from build123d import *

# Parameters (mm, degrees)
SKETCH1_R          = 3.4036
EXTRUDE1_DEPTH     = 1219.2
CUT_EXTRUDE1_DEPTH = 1221.019934263


with BuildPart() as part:
    # Sketch1 → Extrude1 (new, symmetric)
    with BuildSketch(Plane.XY):
        with BuildLine():
            Line((-20, 16.952), (-20, 4.7625))
            ThreePointArc((-20, 4.7625), (-19.776815367, 4.223684633), (-19.238, 4.0005))
            Line((-19.238, 4.0005), (-16.2662, 4.0005))
            ThreePointArc((-16.2662, 4.0005), (-15.727384633, 4.223684633), (-15.5042, 4.7625))
            Line((-15.5042, 4.7625), (-15.5042, 10.485558599))
            ThreePointArc((-15.5042, 10.485558599), (-15.033804775, 11.189554802), (-14.203384633, 11.024373966))
            Line((-14.203384633, 11.024373966), (-8.635059555, 5.456048889))
            ThreePointArc((-8.635059555, 5.456048889), (-7.985348265, 4.483687227), (-7.7572, 3.336708444))
            Line((-7.7572, 3.336708444), (-7.7572, -3.336708444))
            ThreePointArc((-7.7572, -3.336708444), (-7.985348265, -4.483687227), (-8.635059555, -5.456048889))
            Line((-8.635059555, -5.456048889), (-14.203384633, -11.024373966))
            ThreePointArc((-14.203384633, -11.024373966), (-15.033804775, -11.189554802), (-15.5042, -10.485558599))
            Line((-15.5042, -10.485558599), (-15.5042, -4.7625))
            ThreePointArc((-15.5042, -4.7625), (-15.727384633, -4.223684633), (-16.2662, -4.0005))
            Line((-16.2662, -4.0005), (-19.238, -4.0005))
            ThreePointArc((-19.238, -4.0005), (-19.776815367, -4.223684633), (-20, -4.7625))
            Line((-20, -4.7625), (-20, -16.952))
            ThreePointArc((-20, -16.952), (-19.107261469, -19.107261469), (-16.952, -20))
            Line((-16.952, -20), (-4.7625, -20))
            ThreePointArc((-4.7625, -20), (-4.223684633, -19.776815367), (-4.0005, -19.238))
            Line((-4.0005, -19.238), (-4.0005, -16.2662))
            ThreePointArc((-4.0005, -16.2662), (-4.223684633, -15.727384633), (-4.7625, -15.5042))
            Line((-4.7625, -15.5042), (-10.485558599, -15.5042))
            ThreePointArc((-10.485558599, -15.5042), (-11.189554802, -15.033804775), (-11.024373966, -14.203384633))
            Line((-11.024373966, -14.203384633), (-5.456048889, -8.635059555))
            ThreePointArc((-5.456048889, -8.635059555), (-4.483687227, -7.985348265), (-3.336708444, -7.7572))
            Line((-3.336708444, -7.7572), (3.336708444, -7.7572))
            ThreePointArc((3.336708444, -7.7572), (4.483687227, -7.985348265), (5.456048889, -8.635059555))
            Line((5.456048889, -8.635059555), (11.024373966, -14.203384633))
            ThreePointArc((11.024373966, -14.203384633), (11.189554802, -15.033804775), (10.485558599, -15.5042))
            Line((10.485558599, -15.5042), (4.7625, -15.5042))
            ThreePointArc((4.7625, -15.5042), (4.223684633, -15.727384633), (4.0005, -16.2662))
            Line((4.0005, -16.2662), (4.0005, -19.238))
            ThreePointArc((4.0005, -19.238), (4.223684633, -19.776815367), (4.7625, -20))
            Line((4.7625, -20), (16.952, -20))
            ThreePointArc((16.952, -20), (19.107261469, -19.107261469), (20, -16.952))
            Line((20, -16.952), (20, -4.7625))
            ThreePointArc((20, -4.7625), (19.776815367, -4.223684633), (19.238, -4.0005))
            Line((19.238, -4.0005), (16.2662, -4.0005))
            ThreePointArc((16.2662, -4.0005), (15.727384633, -4.223684633), (15.5042, -4.7625))
            Line((15.5042, -4.7625), (15.5042, -10.485558599))
            ThreePointArc((15.5042, -10.485558599), (15.033804775, -11.189554802), (14.203384633, -11.024373966))
            Line((14.203384633, -11.024373966), (8.635059555, -5.456048889))
            ThreePointArc((8.635059555, -5.456048889), (7.985348265, -4.483687227), (7.7572, -3.336708444))
            Line((7.7572, -3.336708444), (7.7572, 3.336708444))
            ThreePointArc((7.7572, 3.336708444), (7.985348265, 4.483687227), (8.635059555, 5.456048889))
            Line((8.635059555, 5.456048889), (14.203384633, 11.024373966))
            ThreePointArc((14.203384633, 11.024373966), (15.033804775, 11.189554802), (15.5042, 10.485558599))
            Line((15.5042, 10.485558599), (15.5042, 4.7625))
            ThreePointArc((15.5042, 4.7625), (15.727384633, 4.223684633), (16.2662, 4.0005))
            Line((16.2662, 4.0005), (19.238, 4.0005))
            ThreePointArc((19.238, 4.0005), (19.776815367, 4.223684633), (20, 4.7625))
            Line((20, 4.7625), (20, 16.952))
            ThreePointArc((20, 16.952), (19.107261469, 19.107261469), (16.952, 20))
            Line((16.952, 20), (4.7625, 20))
            ThreePointArc((4.7625, 20), (4.223684633, 19.776815367), (4.0005, 19.238))
            Line((4.0005, 19.238), (4.0005, 16.2662))
            ThreePointArc((4.0005, 16.2662), (4.223684633, 15.727384633), (4.7625, 15.5042))
            Line((4.7625, 15.5042), (10.485558599, 15.5042))
            ThreePointArc((10.485558599, 15.5042), (11.189554802, 15.033804775), (11.024373966, 14.203384633))
            Line((11.024373966, 14.203384633), (5.456048889, 8.635059555))
            ThreePointArc((5.456048889, 8.635059555), (4.483687227, 7.985348265), (3.336708444, 7.7572))
            Line((3.336708444, 7.7572), (-3.336708444, 7.7572))
            ThreePointArc((-3.336708444, 7.7572), (-4.483687227, 7.985348265), (-5.456048889, 8.635059555))
            Line((-5.456048889, 8.635059555), (-11.024373966, 14.203384633))
            ThreePointArc((-11.024373966, 14.203384633), (-11.189554802, 15.033804775), (-10.485558599, 15.5042))
            Line((-10.485558599, 15.5042), (-4.7625, 15.5042))
            ThreePointArc((-4.7625, 15.5042), (-4.223684633, 15.727384633), (-4.0005, 16.2662))
            Line((-4.0005, 16.2662), (-4.0005, 19.238))
            ThreePointArc((-4.0005, 19.238), (-4.223684633, 19.776815367), (-4.7625, 20))
            Line((-4.7625, 20), (-16.952, 20))
            ThreePointArc((-16.952, 20), (-19.107261469, 19.107261469), (-20, 16.952))
        make_face()
        with Locations(Location((0, 0, 0), (0, 0, 180))):
            Circle(SKETCH1_R, mode=Mode.SUBTRACT)
    extrude(amount=EXTRUDE1_DEPTH, both=True)

    # Sketch2 → Cut-Extrude1 (cut, through all)
    with BuildSketch(Plane(origin=(20, 0, 0), x_dir=(0, 0, -1), z_dir=(1, 0, 0))):
        Polygon((1219.2, -20), (1179.2, 20), (1219.2, 20), align=None)
        Polygon((1124.496158184, 20), (1084.496158184, -20), (-1219.2, -20), (-1219.2, 20), align=None)
    extrude(amount=-CUT_EXTRUDE1_DEPTH, mode=Mode.SUBTRACT)


solid = part.part
Verification items for the finished model (mm, model axes). A direction names the side the tool comes from. Round coordinates to 2 decimals unless told otherwise and drop trailing zeros. Loops run counter-clockwise (first coordinate to the right, second up) from the corner with the lowest first, then second, coordinate; pieces in that order, holes last. Notation, with made-up numbers: (-28, 45.5) - (7, 45.5) arc R23 cw to (7, 82.5) - close; hole circle Ø2 at (-37, 52.25). An arc over 180 degrees is marked (long way). Use a Markdown table: item, result. Add a question column.
1. Section check A-A, the plane y = 0. Record the boundary of the cut face in (x, z), plus the area to 3 significant figures.
2. Gauge pin test, flat ends, axial feed: pin 1 (2 mm diameter, centred on x = -8, y = -2.5, fed in from +Z); pin 2 (3 mm diameter, centred on x = 9.5, y = 11, fed in from -Z); pin 3 (2.5 mm diameter, centred on y = -18.5, z = -1120, fed in from -X). Record the tip position at first contact, or that the pin passes through.
3. Release check for a two-part mould opening along X. For faces 4 (the face through (0, 7.757, -1151)), 5 (the face through (-19.083, 19.131, -1151.422)), 6 (the face through (18, -4, -1151)) record: released by +X, released by -X, zero draft, split by the parting line, or undercut.
4. Section check B-B, the plane x = 0. Record the boundary of the cut face in (y, z), plus the area to 3 significant figures.
5. Access from +Z, -Z, +X, -X, +Y, -Y to the whole of each face (thin tool, end or side, straight path). Record for faces 1 (the face through (0, -7.757, -1151)), 2 (the face through (8.2, -11.38, -1150.99)), 3 (the face through (4, 18, -1151)).
6. Thickness scan on probe 1 along Y at (x, z) = (0, -1163); probe 2 along Y at (x, z) = (9, -1156); probe 3 along X at (y, z) = (17, -1130.5). Record the ranges inside material, lowest first. Write a range as [from, to].
Checks:
| question | item | result |
|---|---|---|
| 1 | outline | (-7.76, -1199.2) - (-3.4, -1199.2) - (-3.4, -1104.5) - (-7.76, -1104.5) - close; (3.4, -1199.2) - (7.76, -1199.2) - (7.76, -1104.5) - (3.4, -1104.5) - close |
| 1 | area | 825 mm^2 |
| 2 | pin 1 | stops at z = -1101.03 |
| 2 | pin 2 | stops at z = -1189.7 |
| 2 | pin 3 | stops at x = -19.99 |
| 3 | face 4 | undercut |
| 3 | face 5 | released by -X |
| 3 | face 6 | zero draft |
| 4 | outline | (-7.76, -1206.96) - (-3.4, -1202.6) - (-3.4, -1101.09) - (-7.76, -1096.74) - close; (3.4, -1195.8) - (7.76, -1191.44) - (7.76, -1112.25) - (3.4, -1107.9) - close |
| 4 | area | 825 mm^2 |
| 5 | face 1 | +Z, -Z, -Y |
| 5 | face 2 | +Z, -Z |
| 5 | face 3 | +Z, -Z, +Y |
| 6 | probe 1 | y = [-7.76, -3.4], [3.4, 7.76] |
| 6 | probe 2 | y = [-20, -15.5], [-12.18, -5.82], [5.82, 12.18], [15.5, 20] |
| 6 | probe 3 | x = [-20, -4], [4, 20] |
